Check sheet for the modelled part. Datum: model origin and axes. Units: mm. Give positions to 0.01 mm unless a question says otherwise; leave off trailing zeros. Order: outer loops, then holes, each group sorted by start corner. A loop starts at its lowest first (then second) coordinate and runs counter-clockwise, first axis right, second up. Notation, with made-up numbers: (11.5, 14) -> (21.5, 14) arc R28 ccw to (21.5, 45) -> close; hole circle Ø1 at (-34, 79.25). An arc over 180 degrees is marked (long way). One line per question, with ' | ' between items.
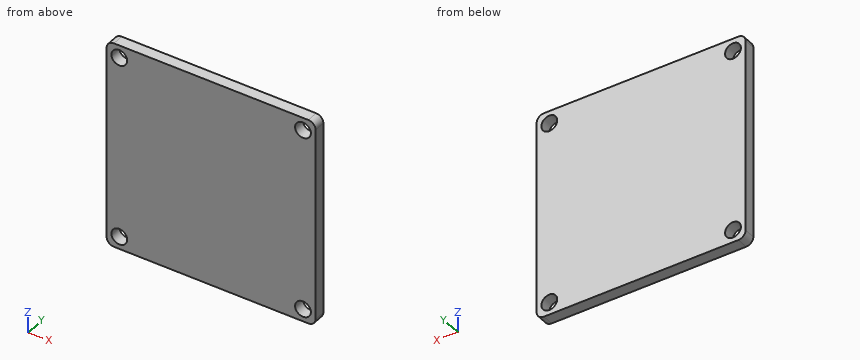
```python
from build123d import *

# Parameters (mm, degrees)
SKIZZE1_W                       = 29
SKIZZE1_H                       = 29
SKIZZE1_R                       = 1.1
AUFSATZ_LINEAR_AUSTRAGEN1_DEPTH = 1.6
VERRUNDUNG1_R                   = 1


with BuildPart() as part:
    # Skizze1 → Aufsatz-Linear austragen1 (new body)
    with BuildSketch(Plane(origin=(0, 0, 0), x_dir=(1, 0, 0), z_dir=(0, 1, 0))):
        Rectangle(SKIZZE1_W, SKIZZE1_H)
        with Locations((-12.75, 12.75)):
            Circle(SKIZZE1_R, mode=Mode.SUBTRACT)
        with Locations((12.75, 12.75)):
            Circle(SKIZZE1_R, mode=Mode.SUBTRACT)
        with Locations((12.75, -12.75)):
            Circle(SKIZZE1_R, mode=Mode.SUBTRACT)
        with Locations((-12.75, -12.75)):
            Circle(SKIZZE1_R, mode=Mode.SUBTRACT)
    extrude(amount=AUFSATZ_LINEAR_AUSTRAGEN1_DEPTH)

    # Verrundung1
    verrundung1_edges = [part.edges().sort_by_distance(p)[0] for p in [
        (14.5, 0.8, 14.5),
        (-14.5, 0.8, 14.5),
        (-14.5, 0.8, -14.5),
        (14.5, 0.8, -14.5),
    ]]
    fillet(verrundung1_edges, radius=VERRUNDUNG1_R)


solid = part.part
```
Q1. Depth check by flat-ended pin: pin 1 Ø1.8 at (x, z) = (12.75, -12.75) entering from -Y. Enter the tip coordinate at first touch or a pass-through.
Result sheet:
pin 1: passes through
Q2. Thickness scan on line 1 (X direction, y = 0.6, z = -12.75); line 2 (Z direction, x = 12.25, y = 0.15). Record the ranges inside material, lowest first.
Result sheet:
line 1: x = -14.5 to -13.85, -11.65 to 11.65, 13.85 to 14.5 | line 2: z = -14.5 to -13.73, -11.77 to 11.77, 13.73 to 14.5
Q3. Section check C-C (y = 0.3). Enter the section's corners in (x, z).
Result sheet:
outline: (-14.5, -13.5) arc R1 ccw to (-13.5, -14.5) -> (13.5, -14.5) arc R1 ccw to (14.5, -13.5) -> (14.5, 13.5) arc R1 ccw to (13.5, 14.5) -> (-13.5, 14.5) arc R1 ccw to (-14.5, 13.5) -> close; hole circle Ø2.2 at (-12.75, -12.75); hole circle Ø2.2 at (-12.75, 12.75); hole circle Ø2.2 at (12.75, -12.75); hole circle Ø2.2 at (12.75, 12.75)
Q4. Section check B-B (z = -12.75). Enter the section's corners in (x, y).
Result sheet:
outline: (-14.5, 0) -> (-13.85, 0) -> (-13.85, 1.6) -> (-14.5, 1.6) -> close; (-11.65, 0) -> (11.65, 0) -> (11.65, 1.6) -> (-11.65, 1.6) -> close; (13.85, 0) -> (14.5, 0) -> (14.5, 1.6) -> (13.85, 1.6) -> close
Q5. Section check A-A (x = 12.75). Enter the section's corners in (y, z), and give its area (3 significant figures).
Result sheet:
outline: (0, -14.5) -> (1.6, -14.5) -> (1.6, -13.85) -> (0, -13.85) -> close; (0, -11.65) -> (1.6, -11.65) -> (1.6, 11.65) -> (0, 11.65) -> close; (0, 13.85) -> (1.6, 13.85) -> (1.6, 14.5) -> (0, 14.5) -> close | area: 39.4 mm2
